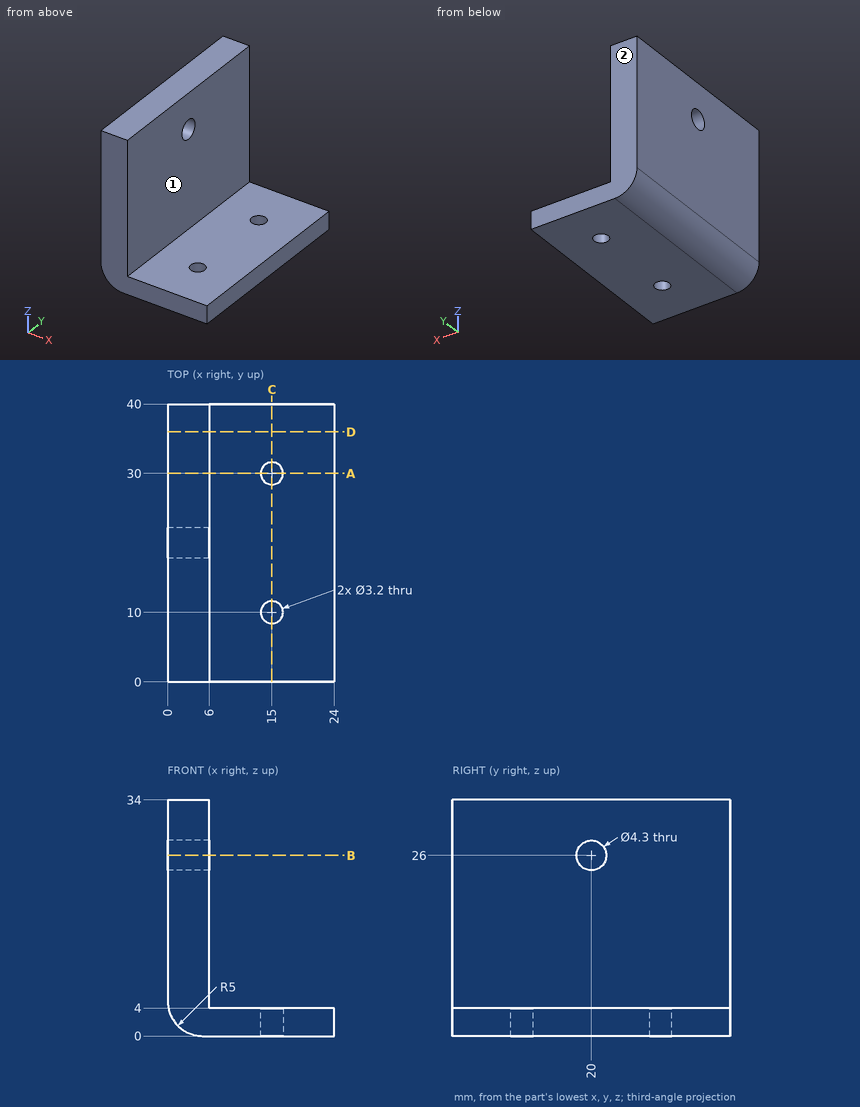
Drawing for the job (mm, zero at the part's lowest x, y, z). A direction names the side the tool comes from. Round coordinates to 2 decimals unless told otherwise and drop trailing zeros. Write each loop counter-clockwise with the first axis right and the second up, starting at its lowest first coordinate (ties: lowest second). Pieces come first, ordered by that corner, then holes. Notation, with made-up numbers: M 40,87.25 L 89,87.25 A27 ccw 89,109.25 Z; hole C 31,53 d10. An arc over 180 degrees is marked long. One line per question, with ' | ' between items.
1. Cut at C-C on x = 15. Write the cut outline in (y, z), and give its area (3 significant figures).
Working result:
outline: M 0,0 L 8.4,0 L 8.4,4 L 0,4 Z; M 11.6,0 L 28.4,0 L 28.4,4 L 11.6,4 Z; M 31.6,0 L 40,0 L 40,4 L 31.6,4 Z | area: 134 mm2
2. Cut at A-A on y = 30. Write the cut outline in (x, z), and give its area (3 significant figures).
Working result:
outline: M 0,5 A5 ccw 5,0 L 13.4,0 L 13.4,4 L 6,4 L 6,34 L 0,34 Z; M 16.6,0 L 24,0 L 24,4 L 16.6,4 Z | area: 258 mm2
3. Which spindle directions (+Z, -Z, +X, -X, +Y, -Y) get a long thin tool onto all of the face, cutting with end or side? Do the marked faces 1 and 2. Say none if no direction does.
Working result:
face 1: +Z, +X, +Y, -Y | face 2: +Z, -Z, +X, -X, +Y
4. Probe L1, parallel to Y at x = 15, z = 1.45; L2, parallel to Z at x = 12.5, y = 18.5; L3, parallel to X at y = 33, z = 14. List the from-to ranges inside material, lowest first. Write a range as from..to.
Working result:
L1: 0..8.4, 11.6..28.4, 31.6..40 | L2: 0..4 | L3: 0..6
5. Cut at B-B on z = 26. Write the cut outline in (x, y), and give its area (3 significant figures).
Working result:
outline: M 0,0 L 6,0 L 6,17.85 L 0,17.85 Z; M 0,22.15 L 6,22.15 L 6,40 L 0,40 Z | area: 214 mm2
6. Pin check, flat tips, straight feed: pin 1 Ø10 at (x, y) = (15.5, 30.5) entering from +Z; pin 2 Ø4 at (y, z) = (30, 22) entering from +X; pin 3 Ø4 at (y, z) = (20, 26) entering from +X. Stop position of each tip, or through.
Working result:
pin 1: z = 4 | pin 2: x = 6 | pin 3: through
7. Cut at D-D on y = 36. Write the cut outline in (x, z), and give its area (3 significant figures).
Working result:
outline: M 0,5 A5 ccw 5,0 L 24,0 L 24,4 L 6,4 L 6,34 L 0,34 Z | area: 271 mm2
